```python
from build123d import *

# Parameters (mm, degrees)
EXTRUSION1_DEPTH = 5
ESQUISSE6_R      = 0.25


with BuildPart() as part:
    # Esquisse2 → Extrusion1 (new body)
    with BuildSketch(Plane(origin=(0, 0, 0), x_dir=(1, 0, 0), z_dir=(0, 1, 0))):
        with BuildLine():
            Line((-2.078460969, -1.2), (2.078460969, -1.2))
            ThreePointArc((2.078460969, -1.2), (0, 2.4), (-2.078460969, -1.2))
        make_face()
    extrude(amount=EXTRUSION1_DEPTH)

    # Balayage1: sweep along a path in Esquisse8
    with BuildLine(Plane(origin=(0, 0, 0), x_dir=(0, 0, -1), z_dir=(1, 0, 0))) as balayage1_path:
        Line((0, 0), (0, -4))
        ThreePointArc((0, -4), (-0.292893219, -4.707106781), (-1, -5))
        Line((-1, -5), (-4.578130226, -5))
    # Esquisse6 → Balayage1 (sweep)
    with BuildSketch(Plane.XZ):
        Circle(ESQUISSE6_R)
        with Locations((1.4, 0)):
            Circle(ESQUISSE6_R)
        with Locations((-1.4, 0)):
            Circle(ESQUISSE6_R)
    sweep(path=balayage1_path.line)


solid = part.part
```
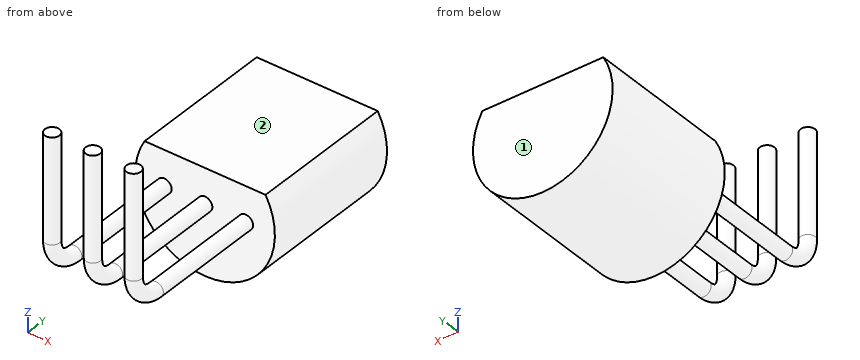
The model under review builds one solid part; all positions refer to its coordinate system, in mm. Face numbers are marked on the shaded views. A direction names the side the tool comes from. Give positions to 0.01 mm unless a question says otherwise; leave off trailing zeros. Write each loop counter-clockwise with the first axis right and the second up, starting at its lowest first coordinate (ties: lowest second). Pieces come first, ordered by that corner, then holes.
(1) Consider section B-B, the plane z = 1.5. Give the boundary of the cut face in (x, y).
(2) Consider section A-A, the plane x = 0. Give the boundary of the cut face in (y, z).
(3) Tool access review of the marked faces 1 and 2: name each direction out of +Z, -Z, +X, -X, +Y, -Y from which nothing blocks a thin tool from reaching the whole face with its end or side.
(4) For P1, Ø2, axis at x = 0, z = 2.5, coming from the +Y side; P2, Ø2, axis at y = -4, z = 0.5, coming from the -X side, all flat-tipped, find the tip position at first contact; note any pin that passes through.
(5) Consider section D-D, the plane y = 2. Give the boundary of the cut face in (x, z).
(6) To check wall thickness, follow L1, parallel to Y at x = 1.85, z = 0.5; L2, parallel to Z at x = -1.1, y = 3.5; L3, parallel to X at y = 4, z = -0.25. State the ranges of each line that lie inside material, in increasing order.
(7) Consider section C-C, the plane y = -0.5. Give the boundary of the cut face in (x, z).
Returned:
1. outline: circle Ø0.5 at (-1.4, -5); circle Ø0.5 at (0, -5); circle Ø0.5 at (1.4, -5)
2. outline: (-5.25, 1) arc R1.25 ccw to (-4, -0.25) - (0, -0.25) - (0, -2.4) - (5, -2.4) - (5, 1.2) - (0, 1.2) - (0, 0.25) - (-4, 0.25) arc R0.75 cw to (-4.75, 1) - (-4.75, 4.58) - (-5.25, 4.58) - close
3. face 1: +Z, -Z, +X, -X, +Y
3. face 2: +Z, +X, -X, +Y
4. P1: stops at y = -4.75
4. P2: stops at x = -1.65
5. outline: (-2.08, 1.2) arc R2.4 ccw (long way) to (2.08, 1.2) - close
6. L1: y = 0 to 5
6. L2: z = -2.13 to 1.2
6. L3: x = -2.39 to 2.39
7. outline: circle Ø0.5 at (-1.4, 0); circle Ø0.5 at (0, 0); circle Ø0.5 at (1.4, 0)
